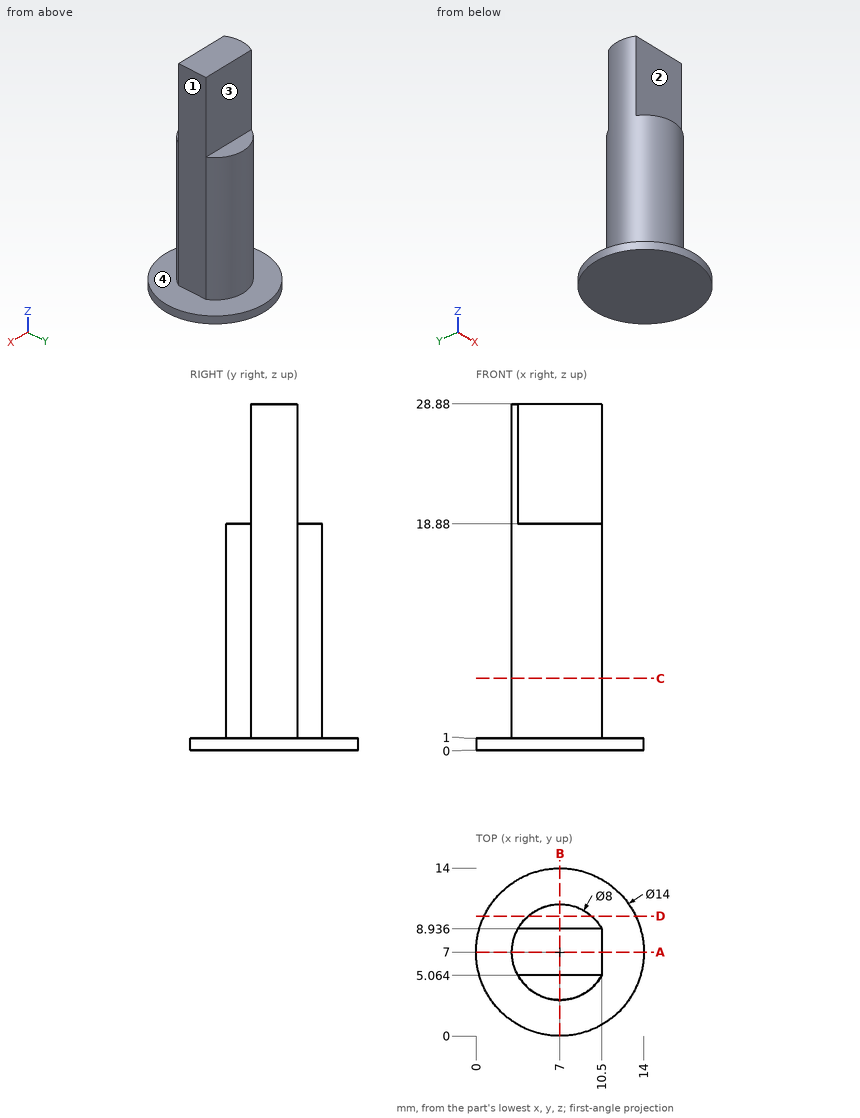
Could you check a few things on this drawing? It's one solid part, dimensions in mm from its lowest x, y, z. A direction names the side the tool comes from. Coordinates: 2 decimals unless noted, no trailing zeros. Loops run counter-clockwise (first coordinate to the right, second up) from the corner with the lowest first, then second, coordinate; pieces in that order, holes last.
1. Imagine slicing it at B-B (x = 7). Please give me the cut outline in (y, z).
2. I need wall thicknesses on L1, parallel to Z at x = 11.5, y = 9; L2, parallel to Y at x = 8.25, z = 24.25; L3, parallel to Z at x = 7.25, y = 3.75. Which ranges of each line are inside material? Lowest first, please.
3. For P1, Ø6, axis at y = 9, z = 6, coming from the +X side; P2, Ø8, axis at y = 4.5, z = 26, coming from the -X side; P3, Ø4, axis at y = 3.5, z = 22.5, coming from the -X side, each with a flat end and sliding along its axis, tell me the tip position at first contact or that it passes through.
4. For the marked faces 1, 2, 3 and 4, which set-ups out of +Z, -Z, +X, -X, +Y, -Y let a thin tool reach every point of the face, with its end or its side?
5. Imagine slicing it at C-C (z = 6). Please give me the cut outline in (x, y).
6. Imagine slicing it at D-D (y = 10). Please give me the cut outline in (x, z) (1 decimal), and give its area (3 significant figures).
7. Imagine slicing it at A-A (y = 7). Please give me the cut outline in (x, z).
Computed values:
1. outline: (0, 0) - (14, 0) - (14, 1) - (11, 1) - (11, 18.88) - (8.94, 18.88) - (8.94, 28.88) - (5.06, 28.88) - (5.06, 18.88) - (3, 18.88) - (3, 1) - (0, 1) - close
2. L1: z = 0 to 1
2. L2: y = 5.06 to 8.94
2. L3: z = 0 to 18.88
3. P1: stops at x = 10.5
3. P2: stops at x = 3
3. P3: stops at x = 3.29
4. face 1: +Z, +X, +Y, -Y
4. face 2: +Z, +X, -X, -Y
4. face 3: +Z, +X, -X, +Y
4. face 4: +Z
5. outline: (10.5, 5.06) - (10.5, 8.94) arc R4 ccw (long way) to start
6. outline: (0.7, 0) - (13.3, 0) - (13.3, 1) - (9.6, 1) - (9.6, 18.9) - (4.4, 18.9) - (4.4, 1) - (0.7, 1) - close
6. area: 107 mm2
7. outline: (0, 0) - (14, 0) - (14, 1) - (10.5, 1) - (10.5, 28.88) - (3, 28.88) - (3, 1) - (0, 1) - close
